The listing builds one solid part. Answer for the finished solid, in the listing's coordinates (mm). A direction names the side the tool comes from. Round coordinates to 2 decimals unless told otherwise and drop trailing zeros. Loops run counter-clockwise (first coordinate to the right, second up) from the corner with the lowest first, then second, coordinate; pieces in that order, holes last. Notation, with made-up numbers: (63.5, 81.5) - (84.5, 81.5) arc R19 cw to (84.5, 114.5) - close; hole circle Ø2 at (15.5, -6.5). An arc over 180 degrees is marked (long way). One line per question, with ' | ' between items. Start each with the question number.
from build123d import *

# Parameters (mm, degrees)
SKETCH_1_W          = 33
SKETCH_1_H          = 80
EXTRUDE_1_DEPTH     = 8
SKETCH_2_W          = 15
SKETCH_2_H          = 10
CUT_EXTRUDE_1_DEPTH = 45.002840817
SKETCH_3_R          = 1.5
CUT_EXTRUDE_2_DEPTH = 45.002840817
SKETCH_4_R          = 1.5
CUT_EXTRUDE_3_DEPTH = 53.469038489
FILLET_2_R          = 1
SKETCH_5_R          = 1.5
CUT_EXTRUDE_4_DEPTH = 45.002840817
SKETCH_7_W          = 15
SKETCH_7_H          = 12
CUT_EXTRUDE_5_DEPTH = 45.002840817
FILLET_3_R          = 3
SKETCH_8_R          = 3
CUT_EXTRUDE_6_DEPTH = 3.5


with BuildPart() as part:
    # 草图1 → 凸台-拉伸1 (new body)
    with BuildSketch(Plane.XY):
        Rectangle(SKETCH_1_W, SKETCH_1_H)
    extrude(amount=EXTRUDE_1_DEPTH)

    # 草图2 → 切除-拉伸1 (cut, through all)
    with BuildSketch(Plane.XY.offset(8)):
        with Locations((0, 35)):
            Rectangle(SKETCH_2_W, SKETCH_2_H)
        with Locations((0, -35)):
            Rectangle(SKETCH_2_W, SKETCH_2_H)
    extrude(amount=-CUT_EXTRUDE_1_DEPTH, mode=Mode.SUBTRACT)

    # 草图3 → 切除-拉伸2 (cut, through all)
    with BuildSketch(Plane.XY.offset(8)):
        with Locations((11.5, 22)):
            Circle(SKETCH_3_R)
        with Locations((11.5, 30)):
            Circle(SKETCH_3_R)
        with Locations(Location((11.5, -30, 0), (0, 0, 180))):
            Circle(SKETCH_3_R)
        with Locations(Location((11.5, -22, 0), (0, 0, 180))):
            Circle(SKETCH_3_R)
        with Locations((-11.5, -22)):
            Circle(SKETCH_3_R)
        with Locations((-11.5, -30)):
            Circle(SKETCH_3_R)
        with Locations(Location((-11.5, 30, 0), (0, 0, 180))):
            Circle(SKETCH_3_R)
        with Locations(Location((-11.5, 22, 0), (0, 0, 180))):
            Circle(SKETCH_3_R)
    extrude(amount=-CUT_EXTRUDE_2_DEPTH, mode=Mode.SUBTRACT)

    # 草图4 → 切除-拉伸3 (cut, through all)
    with BuildSketch(Plane.ZY.offset(16.5)):
        with Locations((5, 36)):
            Circle(SKETCH_4_R)
        with Locations(Location((5, -36, 0), (0, 0, 180))):
            Circle(SKETCH_4_R)
    extrude(amount=-CUT_EXTRUDE_3_DEPTH, mode=Mode.SUBTRACT)

    # 圆角2
    fillet_2_edges = [part.edges().sort_by_distance(p)[0] for p in [
        (7.5, 30, 4),
        (-7.5, 30, 4),
        (-7.5, -30, 4),
        (7.5, -30, 4),
    ]]
    fillet(fillet_2_edges, radius=FILLET_2_R)

    # 草图5 → 切除-拉伸4 (cut, through all)
    with BuildSketch(Plane(origin=(0, 0, 0), x_dir=(-1, 0, 0), z_dir=(0, 0, -1))):
        Circle(SKETCH_5_R)
        with Locations((0, 27)):
            Circle(SKETCH_5_R)
        with Locations(Location((0, -27, 0), (0, 0, 180))):
            Circle(SKETCH_5_R)
    extrude(amount=-CUT_EXTRUDE_4_DEPTH, mode=Mode.SUBTRACT)

    # 草图7 → 切除-拉伸5 (cut, through all)
    with BuildSketch(Plane(origin=(0, 0, 0), x_dir=(-1, 0, 0), z_dir=(0, 0, -1))):
        with Locations((0, 15)):
            Rectangle(SKETCH_7_W, SKETCH_7_H)
        with Locations((0, -15)):
            Rectangle(SKETCH_7_W, SKETCH_7_H)
    extrude(amount=-CUT_EXTRUDE_5_DEPTH, mode=Mode.SUBTRACT)

    # 圆角3
    fillet_3_edges = [part.edges().sort_by_distance(p)[0] for p in [
        (-7.5, 21, 4),
        (-7.5, 9, 4),
        (7.5, 9, 4),
        (7.5, 21, 4),
        (7.5, -21, 4),
        (7.5, -9, 4),
        (-7.5, -9, 4),
        (-7.5, -21, 4),
    ]]
    fillet(fillet_3_edges, radius=FILLET_3_R)

    # 草图8 → 切除-拉伸6 (cut)
    with BuildSketch(Plane(origin=(0, 0, 0), x_dir=(-1, 0, 0), z_dir=(0, 0, -1))):
        with Locations((11.5, 30)):
            Circle(SKETCH_8_R)
        with Locations((-11.5, 30)):
            Circle(SKETCH_8_R)
        with Locations((-11.5, -30)):
            Circle(SKETCH_8_R)
        with Locations((11.5, -30)):
            Circle(SKETCH_8_R)
        Circle(SKETCH_8_R)
    extrude(amount=-CUT_EXTRUDE_6_DEPTH, mode=Mode.SUBTRACT)


solid = part.part
(1) Determine the mould class of faces 1 (the cylindrical face through (-0.195, -28.487, 3.944)), 2 (the flat face through (-4, 1, 0)), 3 (the cylindrical face through (-6.6, 20.14, 4.06)), 4 (the flat face through (-12, -40, 4)) for opening direction Y: pulls with the +Y half, pulls with the -Y half, needs draft (parallel to the pull), parting line crosses it, or undercut.
(2) A tool of negligible diameter and unlimited length cuts with its end or side. For faces 5 (the cylindrical face through (13.71, 32.03, 1.73)), 6 (the flat face through (-7.5, 15, 4)), 7 (the flat face through (-12, 40, 4)), from which of +Z, -Z, +X, -X, +Y, -Y can it reach the whole face along a straight path? Write none if from no direction.
(3) Consider L1, parallel to Y at x = 0, z = 1.95; L2, parallel to Y at x = 0, z = 5.5; L3, parallel to Y at x = -14, z = 5. Determine where each line is inside the solid, lowest interval first.
(4) Find section A-A on x = -11.5. Count the separate pieces of the cut face and the enclosed holes in it, plus the area to 3 significant figures.
(5) Find section B-B on y = 17. Write down the section's boundary in (x, z), plus the area to 3 significant figures.
(6) Each of these flat-tipped pins is pushed along its axis until it touches: P1, Ø1, axis at x = 2.5, y = -19, coming from the +Z side; P2, Ø2.5, axis at x = 0, z = 4.5, coming from the -Y side; P3, Ø2.5, axis at x = -1, z = 3, coming from the +Y side; P4, Ø3, axis at x = -5.5, z = 5, coming from the +Y side. Where does it stop, or does it pass through?
Answer below:
1) face 1: undercut | face 2: needs draft | face 3: undercut | face 4: pulls with the -Y half
2) face 5: -Z | face 6: +Z, -Z | face 7: +Z, -Z, +X, -X, +Y
3) L1: -30 to -28.5, -25.5 to -21, -9 to -3, 3 to 9, 21 to 25.5, 28.5 to 30 | L2: -30 to -28.5, -25.5 to -21, -9 to -1.5, 1.5 to 9, 21 to 25.5, 28.5 to 30 | L3: -40 to -37.5, -34.5 to 34.5, 37.5 to 40
4) separate pieces: 5 | enclosed holes: 2 | area: 509 mm2
5) outline: (-16.5, 0) - (-7.5, 0) - (-7.5, 8) - (-16.5, 8) - close; (7.5, 0) - (16.5, 0) - (16.5, 8) - (7.5, 8) - close | area: 144 mm2
6) P1: through | P2: y = -30 | P3: y = 30 | P4: y = 30.13
